Design review of the part built by this model. Coordinates are the model's own, in mm. Coordinates: 2 decimals unless noted, no trailing zeros. Loops run counter-clockwise (first coordinate to the right, second up) from the corner with the lowest first, then second, coordinate; pieces in that order, holes last. Notation, with made-up numbers: (71.5, -9) -> (130.5, -9) arc R13 cw to (130.5, 6) -> close; hole circle Ø2 at (-26.5, 76.25). An arc over 180 degrees is marked (long way). Use a Markdown table: item, result. Add a question column.
Q1. Draft analysis for pull direction X (two halves, no side actions). For faces 1 (the face through (-0.16, 1.97, 13.74)), 2 (the face through (-8.4, 4, -3.8)), 3 (the face through (-3.956, 1.972, -17.816)), state which applies: pulls with the +X half, pulls with the -X half, needs draft (parallel to the pull), parting line crosses it, or undercut.
Q2. For probe 1 along Z at (x, y) = (0, 0.9); probe 2 along X at (y, z) = (1.6, 7); probe 3 along Z at (x, y) = (-12, 3.5), list the stretches that pass through material, from the lowest coordinate up.
Q3. Take a section at B-B on x = -7. Write out the cut boundary in (y, z).
Q4. Take a section at A-A on z = -4. Write out the cut boundary in (x, y).
Q5. Take a section at C-C on y = 3.2. Count the separate pieces of the cut face and the enclosed holes in it, plus the area to 3 significant figures.
Q6. Clearance check with flat-ended pins moving along their axes: pin 1 Ø4 at (x, z) = (11.5, 9) entering from -Y; pin 2 Ø3.5 at (x, z) = (13.38, 7.73) entering from +Y; pin 3 Ø1 at (x, y) = (9, 3) entering from -Z; pin 4 Ø2 at (y, z) = (3, -8.5) entering from +X. State where each tip first meets the part, or that it passes through.
Q7. Take a section at D-D on x = 14.5. Write out the cut boundary in (y, z).
from build123d import *

# Parameters (mm, degrees)
F0_R     = 18.25
F0_R_2   = 1.25
F0_R_3   = 9
F1_DEPTH = 4
F2_R     = 1.825
F3_DEPTH = 25


with BuildPart() as f1:
    # F0 (on Front) → F1 (new body)
    with BuildSketch(Plane.XZ):
        Circle(F0_R)
        with Locations((-7.347316, -10.112712)):
            Circle(F0_R_2, mode=Mode.SUBTRACT)
        with Locations((7.347316, -10.112712)):
            Circle(F0_R_2, mode=Mode.SUBTRACT)
        with Locations((-11.888206, 3.862712)):
            Circle(F0_R_2, mode=Mode.SUBTRACT)
        Circle(F0_R_3, mode=Mode.SUBTRACT)
        with Locations((11.888206, 3.862712)):
            Circle(F0_R_2, mode=Mode.SUBTRACT)
        with Locations((0, 12.5)):
            Circle(F0_R_2, mode=Mode.SUBTRACT)
    extrude(amount=-F1_DEPTH)

    # F2 (on face) → F3 (cut)
    with BuildSketch(Plane(origin=(0, 4, 0), x_dir=(-1, 0, 0), z_dir=(0, 1, 0))):
        with Locations((-13.384261, 7.727407)):
            Circle(F2_R)
        with Locations((13.384261, 7.727407)):
            Circle(F2_R)
        with Locations((0, -15.454813)):
            Circle(F2_R)
    extrude(amount=-F3_DEPTH, mode=Mode.SUBTRACT)


solid = f1.part
Answer list:
| question | item | result |
|---|---|---|
| 1 | face 1 | undercut |
| 1 | face 2 | needs draft |
| 1 | face 3 | parting line crosses it |
| 2 | probe 1 | -18.25 to -17.28, -13.63 to -9, 9 to 11.25, 13.75 to 18.25 |
| 2 | probe 2 | -16.85 to -15.06, -11.71 to -5.66, 5.66 to 11.71, 15.06 to 16.85 |
| 2 | probe 3 | -13.75 to 2.62, 5.11 to 6.54, 8.92 to 13.75 |
| 3 | outline | (0, -16.85) -> (4, -16.85) -> (4, -11.31) -> (0, -11.31) -> close; (0, -8.91) -> (4, -8.91) -> (4, -5.66) -> (0, -5.66) -> close; (0, 5.66) -> (4, 5.66) -> (4, 16.85) -> (0, 16.85) -> close |
| 4 | outline | (-17.81, 0) -> (-8.06, 0) -> (-8.06, 4) -> (-17.81, 4) -> close; (8.06, 0) -> (17.81, 0) -> (17.81, 4) -> (8.06, 4) -> close |
| 5 | separate pieces | 1 |
| 5 | enclosed holes | 9 |
| 5 | area | 736 mm² |
| 6 | pin 1 | y = 0 |
| 6 | pin 2 | through |
| 6 | pin 3 | z = -16.15 |
| 6 | pin 4 | x = 16.64 |
| 7 | outline | (0, -11.08) -> (4, -11.08) -> (4, 6.28) -> (0, 6.28) -> close; (0, 9.17) -> (4, 9.17) -> (4, 11.08) -> (0, 11.08) -> close |
